Autodesk Inventor part; units mm, degrees
ref_plane "YZ Plane" through (0, 0, 0) normal (1, 0, 0) x (0, 1, 0)
ref_plane "XZ Plane" through (0, 0, 0) normal (0, 1, 0) x (-1, 0, 0)
ref_plane "XY Plane" through (0, 0, 0) normal (0, 0, 1) x (1, 0, 0)
sketch "Sketch1" plane through (0, 0, 0) normal (0, 1, 0) x (-1, 0, 0)
  line L0 (0, 0) -> (0, 4.65)
  line L1 (0, 4.65) -> (-5, 4.65)
  line L2 (-5, 4.65) -> (-5, 7.5)
  line L3 (-5, 7.5) -> (25, 7.5)
  line L4 (25, 7.5) -> (25, 0)
  line L5 (25, 0) -> (0, 0) construction
  line L6 (0, 0) -> (0, -4.65)
  line L7 (0, -4.65) -> (-5, -4.65)
  line L8 (-5, -4.65) -> (-5, -7.5)
  line L9 (-5, -7.5) -> (25, -7.5)
  line L10 (25, -7.5) -> (25, 0)
  dimension "d7" = 9.3
  dimension "d8" = 15
  dimension "d9" = 5
  dimension "d10" = 25
extrude "Extrusion1" add sketch "Sketch1" along normal blind 9
sketch "Sketch2" plane through (0, 9, 0) normal (0, 1, 0) x (1, 0, 0)
  line L0 (5, 7.5) -> (-25, 7.5)
  line L1 (-25, 7.5) -> (-25, -7.5)
  line L2 (-25, -7.5) -> (5, -7.5)
  line L3 (-20, 7.5) -> (-20, -7.5)
  point P0 (0, 0)
  dimension "d11" = 5
extrude "Extrusion2" add sketch "Sketch2" along normal blind 5
sketch "Sketch3" plane through (0, 0, 4.65) normal (1, 0, 0) x (0, 0, -1)
  line L0 (9.3, 0) -> (9.3, 9)
  line L1 (0, 9) -> (9.3, 9)
  line L2 (0, 0) -> (0, 9)
  line L3 (0, 4.5) -> (9.3, 4.5) construction
  line L4 (4.65, 9) -> (4.65, 0) construction
  circle A0 centre (4.65, 4.5) radius 1.5
  dimension "d4" = 3
extrude "Extrusion3" cut sketch "Sketch3" against normal blind 15
fillet "Fillet1" radius 2 2 edges at (-10, 0, -7.5) (-10, 0, 7.5)
properties part number "Carcasa (parte 2)"
Model file for the job. Use its own axes, mm. A direction names the side the tool comes from. Give positions to 0.01 mm unless a question says otherwise; leave off trailing zeros. Loops run counter-clockwise (first coordinate to the right, second up) from the corner with the lowest first, then second, coordinate; pieces in that order, holes last. Notation, with made-up numbers: (33.25, -11) - (87.25, -11) arc R18 cw to (87.25, 12) - close; hole circle Ø10 at (42, 39). An arc over 180 degrees is marked (long way). Use one line per item in the form item = value.
(1) Drill centre lines: L1, parallel to Y at x = -7.5, z = 0; L2, parallel to Y at x = -13, z = -3.5; L3, parallel to X at y = 4, z = -1. Where is each one in solid material? Low to high.
Determined:
L1 = 0 to 3, 6 to 9
L2 = 0 to 9
L3 = -25 to -15
(2) 3-axis set-ups, long thin cutter, end or side, ignore diameter. For faces 4 (the face through (-20, 11, 0)), 5 (the face through (-7.4, 4.57, 1.5)), 6 (the face through (2, 4, 4.65)): which of +Z, -Z, +X, -X, +Y, -Y reach the whole face in a straight line?
Determined:
face_4 = +Z, -Z, +X, +Y
face_5 = +X
face_6 = +X, +Y, -Y
(3) Cut at A-A (x = -1). Give the cut face in (y, z), then the cut area to 3 significant figures.
Determined:
outline = (0, -5.5) arc R2 ccw to (2, -7.5) - (9, -7.5) - (9, 7.5) - (2, 7.5) arc R2 ccw to (0, 5.5) - close; hole circle Ø3 at (4.5, 0)
area = 126 mm^2
(4) Drop flat-ended pins along their axis: P1, Ø1.5, axis at y = 12.5, z = 2.5, coming from the +X side; P2, Ø4, axis at y = 4.5, z = 0, coming from the +X side; P3, Ø1.5, axis at y = 4, z = -0.5, coming from the +X side. Give the stop position or say it passes through.
Determined:
P1 = -20
P2 = 0
P3 = -15
(5) Cut at B-B (y = 4.5). Give the cut face in (x, z), then the cut area to 4 significant figures.
Determined:
outline = (-25, -7.5) - (5, -7.5) - (5, -4.65) - (0, -4.65) - (0, -1.5) - (-15, -1.5) - (-15, 1.5) - (0, 1.5) - (0, 4.65) - (5, 4.65) - (5, 7.5) - (-25, 7.5) - close
area = 358.5 mm^2
(6) Pull direction Z, two halves, no side cores. Call faces 1 (the face through (-10, 5, 7.5)), 2 (the face through (0, 3, -1)), 3 (the face through (-10, 5, -7.5)): pulls with the +Z half, pulls with the -Z half, needs draft (parallel to the pull), parting line crosses it, or undercut.
Determined:
face_1 = pulls with the +Z half
face_2 = undercut
face_3 = pulls with the -Z half
(7) Cut at C-C (z = 0). Give the cut face in (x, y).
Determined:
outline = (-25, 0) - (0, 0) - (0, 3) - (-15, 3) - (-15, 6) - (0, 6) - (0, 9) - (-20, 9) - (-20, 14) - (-25, 14) - close
(8) Cut at D-D (y = 7.5). Give the cut face in (x, z), then the cut area to 4 significant figures.
Determined:
outline = (-25, -7.5) - (5, -7.5) - (5, -4.65) - (0, -4.65) - (0, 4.65) - (5, 4.65) - (5, 7.5) - (-25, 7.5) - close
area = 403.5 mm^2
